from build123d import *

# Parameters (mm, degrees)
MODEL_W             = 101.6
MODEL_H             = 398.78
BOSS_EXTRUDE1_DEPTH = 6.35
SKETCH1_W           = 6.35
SKETCH1_H           = 10.16
CUT_EXTRUDE1_DEPTH  = 6.35


with BuildPart() as part:
    # Model → Boss-Extrude1 (new body)
    with BuildSketch(Plane.XY):
        with Locations((50.8, 199.39)):
            Rectangle(MODEL_W, MODEL_H)
        with BuildLine():
            Line((83.820574672, 83.411866713), (20.83121403, 87.63))
            ThreePointArc((20.83121403, 87.63), (18.406749642, 85.847345646), (19.385420684, 83.001631833))
            Line((19.385420684, 83.001631833), (91.264206654, 33.239395393))
            ThreePointArc((91.264206654, 33.239395393), (93.888830968, 33.077884107), (95.25, 35.32776356))
            Line((95.25, 35.32776356), (90.076491123, 77.061866713))
            ThreePointArc((90.076491123, 77.061866713), (88.249801524, 81.518855344), (83.820574672, 83.411866713))
        make_face(mode=Mode.SUBTRACT)
        with BuildLine():
            Line((11.034694705, 153.003483907), (6.35, 111.52776356))
            ThreePointArc((6.35, 111.52776356), (7.711169032, 109.277884107), (10.335793346, 109.439395393))
            Line((10.335793346, 109.439395393), (82.214579316, 159.201631833))
            ThreePointArc((82.214579316, 159.201631833), (83.193250358, 162.047345646), (80.76878597, 163.83))
            Line((80.76878597, 163.83), (16.773036865, 158.741826067))
            ThreePointArc((16.773036865, 158.741826067), (12.715416211, 157.061104561), (11.034694705, 153.003483907))
        make_face(mode=Mode.SUBTRACT)
        with BuildLine():
            Line((84.100188096, 235.630146894), (20.83121403, 240.03))
            ThreePointArc((20.83121403, 240.03), (18.406749642, 238.247345646), (19.385420684, 235.401631833))
            Line((19.385420684, 235.401631833), (91.264206654, 185.639395393))
            ThreePointArc((91.264206654, 185.639395393), (93.888830968, 185.477884107), (95.25, 187.72776356))
            Line((95.25, 187.72776356), (90.086811771, 229.280146894))
            ThreePointArc((90.086811771, 229.280146894), (88.354189205, 233.643693703), (84.100188096, 235.630146894))
        make_face(mode=Mode.SUBTRACT)
        with BuildLine():
            Line((16.773036865, 181.402479512), (80.76878597, 176.53))
            ThreePointArc((80.76878597, 176.53), (83.193250358, 178.312654354), (82.214579316, 181.158368167))
            Line((82.214579316, 181.158368167), (10.335793346, 230.920604607))
            ThreePointArc((10.335793346, 230.920604607), (7.711169032, 231.082115893), (6.35, 228.83223644))
            Line((6.35, 228.83223644), (11.910018955, 186.265497422))
            ThreePointArc((11.910018955, 186.265497422), (13.334363923, 182.826824481), (16.773036865, 181.402479512))
        make_face(mode=Mode.SUBTRACT)
        with BuildLine():
            Line((91.264206654, 154.720604607), (19.385420684, 104.958368167))
            ThreePointArc((19.385420684, 104.958368167), (18.406749642, 102.112654354), (20.83121403, 100.33))
            Line((20.83121403, 100.33), (83.725783656, 106.06798896))
            ThreePointArc((83.725783656, 106.06798896), (88.215911716, 107.9278609), (90.075783656, 112.41798896))
            Line((90.075783656, 112.41798896), (95.25, 152.63223644))
            ThreePointArc((95.25, 152.63223644), (93.888830968, 154.882115893), (91.264206654, 154.720604607))
        make_face(mode=Mode.SUBTRACT)
        with BuildLine():
            Line((10.271454318, 305.232761919), (6.35, 263.92776356))
            ThreePointArc((6.35, 263.92776356), (7.711169032, 261.677884107), (10.335793346, 261.839395393))
            Line((10.335793346, 261.839395393), (82.214579316, 311.601631833))
            ThreePointArc((82.214579316, 311.601631833), (83.193250358, 314.447345646), (80.76878597, 316.23))
            Line((80.76878597, 316.23), (16.773036865, 311.734344465))
            ThreePointArc((16.773036865, 311.734344465), (12.175723757, 309.830075026), (10.271454318, 305.232761919))
        make_face(mode=Mode.SUBTRACT)
        with BuildLine():
            Line((88.9, 392.43), (20.83121403, 392.43))
            ThreePointArc((20.83121403, 392.43), (18.406749642, 390.647345646), (19.385420684, 387.801631833))
            Line((19.385420684, 387.801631833), (91.264206654, 338.039395393))
            ThreePointArc((91.264206654, 338.039395393), (93.888830968, 337.877884107), (95.25, 340.12776356))
            Line((95.25, 340.12776356), (95.25, 386.08))
            ThreePointArc((95.25, 386.08), (93.390128061, 390.570128061), (88.9, 392.43))
        make_face(mode=Mode.SUBTRACT)
        with BuildLine():
            Line((16.773036865, 333.700240414), (80.76878597, 328.93))
            ThreePointArc((80.76878597, 328.93), (83.193250358, 330.712654354), (82.214579316, 333.558368167))
            Line((82.214579316, 333.558368167), (10.335793346, 383.320604607))
            ThreePointArc((10.335793346, 383.320604607), (7.711169032, 383.482115893), (6.35, 381.23223644))
            Line((6.35, 381.23223644), (11.254237586, 339.219039692))
            ThreePointArc((11.254237586, 339.219039692), (12.870656471, 335.316659298), (16.773036865, 333.700240414))
        make_face(mode=Mode.SUBTRACT)
        with BuildLine():
            Line((16.773036865, 28.615297102), (80.76878597, 24.13))
            ThreePointArc((80.76878597, 24.13), (83.193250358, 25.912654354), (82.214579316, 28.758368167))
            Line((82.214579316, 28.758368167), (10.335793346, 78.520604607))
            ThreePointArc((10.335793346, 78.520604607), (7.711169032, 78.682115893), (6.35, 76.43223644))
            Line((6.35, 76.43223644), (10.423036865, 34.965297102))
            ThreePointArc((10.423036865, 34.965297102), (12.282908804, 30.475169041), (16.773036865, 28.615297102))
        make_face(mode=Mode.SUBTRACT)
        with BuildLine():
            Line((91.264206654, 307.120604607), (19.385420684, 257.358368167))
            ThreePointArc((19.385420684, 257.358368167), (18.406749642, 254.512654354), (20.83121403, 252.73))
            Line((20.83121403, 252.73), (84.309327563, 258.27471682))
            ThreePointArc((84.309327563, 258.27471682), (88.4366297, 260.326932153), (90.102540158, 264.62471682))
            Line((90.102540158, 264.62471682), (95.25, 305.03223644))
            ThreePointArc((95.25, 305.03223644), (93.888830968, 307.282115893), (91.264206654, 307.120604607))
        make_face(mode=Mode.SUBTRACT)
    extrude(amount=BOSS_EXTRUDE1_DEPTH)

    # Sketch1 → Cut-Extrude1 (cut)
    with BuildSketch(Plane.XY.offset(6.35)):
        with Locations((98.425, 19.05)):
            Rectangle(SKETCH1_W, SKETCH1_H)
        with Locations((3.175, 95.25)):
            Rectangle(SKETCH1_W, SKETCH1_H)
        with Locations((98.425, 171.45)):
            Rectangle(SKETCH1_W, SKETCH1_H)
        with Locations((3.175, 171.45)):
            Rectangle(SKETCH1_W, SKETCH1_H)
        with Locations((98.425, 247.65)):
            Rectangle(SKETCH1_W, SKETCH1_H)
        with Locations((3.175, 323.85)):
            Rectangle(SKETCH1_W, SKETCH1_H)
        with Locations((3.175, 19.05)):
            Rectangle(SKETCH1_W, SKETCH1_H)
        with Locations((98.425, 95.25)):
            Rectangle(SKETCH1_W, SKETCH1_H)
        with Locations((3.175, 247.65)):
            Rectangle(SKETCH1_W, SKETCH1_H)
        with Locations((98.425, 323.85)):
            Rectangle(SKETCH1_W, SKETCH1_H)
    extrude(amount=-CUT_EXTRUDE1_DEPTH, mode=Mode.SUBTRACT)


solid = part.part
Verification items for the finished model (mm, model axes). A direction names the side the tool comes from. Give positions to 0.01 mm unless a question says otherwise; leave off trailing zeros. Order: outer loops, then holes, each group sorted by start corner. A loop starts at its lowest first (then second) coordinate and runs counter-clockwise, first axis right, second up. Notation, with made-up numbers: (58.5, 77.25) -> (90.5, 77.25) arc R17 cw to (90.5, 99.25) -> close; hole circle Ø8 at (23, 70). An arc over 180 degrees is marked (long way). Answer as CSV lines item,"result".
Q1. Access from +Z, -Z, +X, -X, +Y, -Y to the whole of each face (thin tool, end or side, straight path). Record for faces 5 (the flat face through (3, 242.57, 3)), 6 (the flat face through (101.6, 57, 3)), 7 (the flat face through (95.25, 19, 3)), 8 (the cylindrical face through (88.17, 107.88, 3.13)).
Solutions:
face 5,"+Z, -Z, -X"
face 6,"+Z, -Z, +X, +Y, -Y"
face 7,"+Z, -Z, +X"
face 8,"+Z, -Z"
Q2. Sectioned sample at B-B on z = 1. Count the separate pieces of the cut face and the enclosed holes in it, plus the area to 3 significant figures.
Solutions:
separate pieces,"1"
enclosed holes,"10"
area,"19,600 mm²"
Q3. Sectioned sample at C-C on y = 125. Record the cut outline in (x, z).
Solutions:
outline,"(0, 0) -> (7.87, 0) -> (7.87, 6.35) -> (0, 6.35) -> close; (32.81, 0) -> (48.33, 0) -> (48.33, 6.35) -> (32.81, 6.35) -> close; (91.69, 0) -> (101.6, 0) -> (101.6, 6.35) -> (91.69, 6.35) -> close"
Q4. Scan lines: probe 1 along X at (y, z) = (214.5, 4.5); probe 2 along X at (y, z) = (212, 5.5); probe 3 along Y at (x, z) = (16, 2.25). Record each from-to range of solid material in increasing order.
Solutions:
probe 1,"x = 0 to 8.22, 34.05 to 49.58, 91.92 to 101.6"
probe 2,"x = 0 to 8.55, 37.67 to 53.19, 92.23 to 101.6"
probe 3,"y = 0 to 28.66, 74.6 to 113.36, 158.69 to 181.46, 227 to 265.76, 311.69 to 333.75, 379.4 to 398.78"
Q5. Sectioned sample at A-A on y = 287.5. Record the cut outline in (x, z).
Solutions:
outline,"(0, 0) -> (8.59, 0) -> (8.59, 6.35) -> (0, 6.35) -> close; (47.4, 0) -> (62.92, 0) -> (62.92, 6.35) -> (47.4, 6.35) -> close; (93.02, 0) -> (101.6, 0) -> (101.6, 6.35) -> (93.02, 6.35) -> close"
Q6. Release check for a two-part mould opening along Y. For faces 1 (the flat face through (50, 0, 3)), 2 (the flat face through (95.25, 363, 3)), 3 (the cylindrical face through (88.392, 260.278, 3.131)), 4 (the flat face through (0, 7, 3)) record: +Y half, -Y half, draft (parallel to the pull), parting line (faces both ways), or undercut.
Solutions:
face 1,"-Y half"
face 2,"undercut"
face 3,"undercut"
face 4,"draft"
